Geometry check sheet. Reference: drawing and pictorial views, mm from the part's lowest x, y, z. Round coordinates to 2 decimals unless told otherwise and drop trailing zeros. Order: outer loops, then holes, each group sorted by start corner. A loop starts at its lowest first (then second) coordinate and runs counter-clockwise, first axis right, second up.
Q1. Depth check by flat-ended pin: P1, Ø2, axis at y = 14, z = 4, coming from the -X side; P2, Ø3.5, axis at x = 97.5, z = 6, coming from the +Y side; P3, Ø1, axis at y = 45, z = 0.5, coming from the -X side; P4, Ø2.5, axis at x = 97.5, z = 6, coming from the +Y side. Enter the tip coordinate at first touch or a pass-through.
Q2. Scan lines: probe 1 along Y at (x, z) = (89.5, 6); probe 2 along Z at (x, y) = (97.5, 35.8); probe 3 along Z at (x, y) = (98, 29.5). Record each from-to range of solid material in increasing order.
Q3. Cross-section at A-A on x = 97.5. Record the cut outline in (y, z), then the cut area to 3 significant figures.
Q4. Mould release check, pull along Y, two halves, no side actions. Record for the marked faces 1, 2 and 3: +Y half, -Y half, draft (parallel to the pull), parting line (faces both ways), or undercut.
Q5. Cross-section at B-B on z = 9. Record the cut outline in (x, y).
Q6. Cross-section at D-D on x = 27.5. Record the cut outline in (y, z).
Q7. Cross-section at C-C on y = 45. Record the cut outline in (x, z), then the cut area to 3 significant figures.
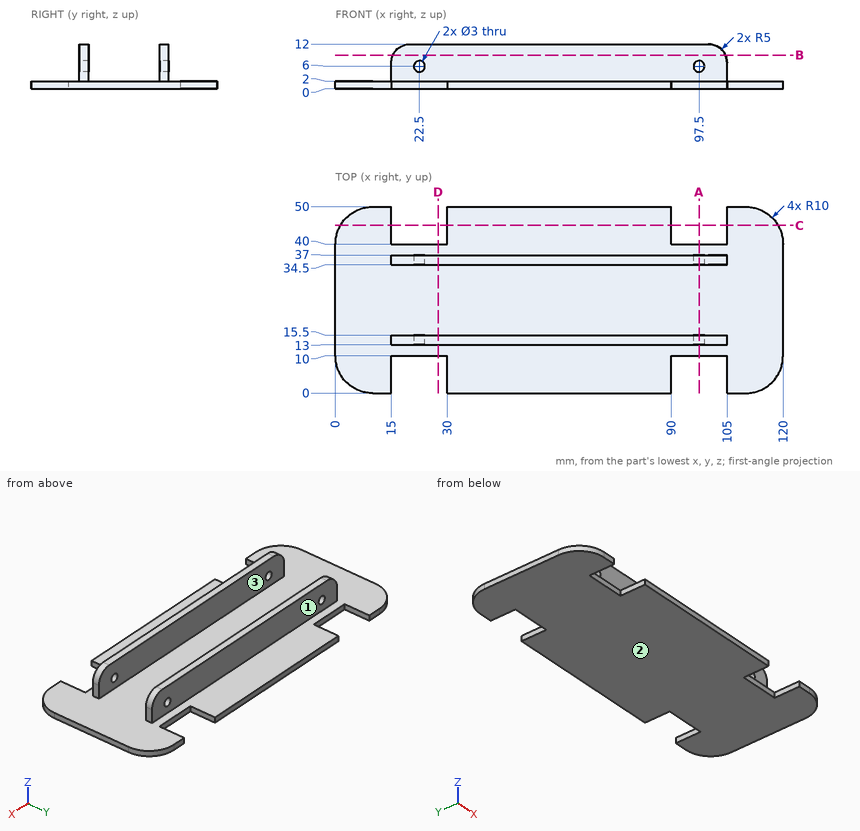
Results found:
1. P1: stops at x = 15
1. P2: stops at y = 37
1. P3: stops at x = 1.07
1. P4: passes through
2. probe 1: y = 13 to 15.5, 34.5 to 37
2. probe 2: z = 0 to 4.5, 7.5 to 12
2. probe 3: z = 0 to 2
3. outline: (10, 0) - (40, 0) - (40, 2) - (37, 2) - (37, 4.5) - (34.5, 4.5) - (34.5, 2) - (15.5, 2) - (15.5, 4.5) - (13, 4.5) - (13, 2) - (10, 2) - close; (13, 7.5) - (15.5, 7.5) - (15.5, 12) - (13, 12) - close; (34.5, 7.5) - (37, 7.5) - (37, 12) - (34.5, 12) - close
3. area: 95.0 mm2
4. face 1: +Y half
4. face 2: draft
4. face 3: undercut
5. outline: (15.42, 13) - (104.58, 13) - (104.58, 15.5) - (15.42, 15.5) - close; (15.42, 34.5) - (104.58, 34.5) - (104.58, 37) - (15.42, 37) - close
6. outline: (10, 0) - (40, 0) - (40, 2) - (37, 2) - (37, 12) - (34.5, 12) - (34.5, 2) - (15.5, 2) - (15.5, 12) - (13, 12) - (13, 2) - (10, 2) - close
7. outline: (1.34, 0) - (15, 0) - (15, 2) - (1.34, 2) - close; (30, 0) - (90, 0) - (90, 2) - (30, 2) - close; (105, 0) - (118.66, 0) - (118.66, 2) - (105, 2) - close
7. area: 175 mm2
